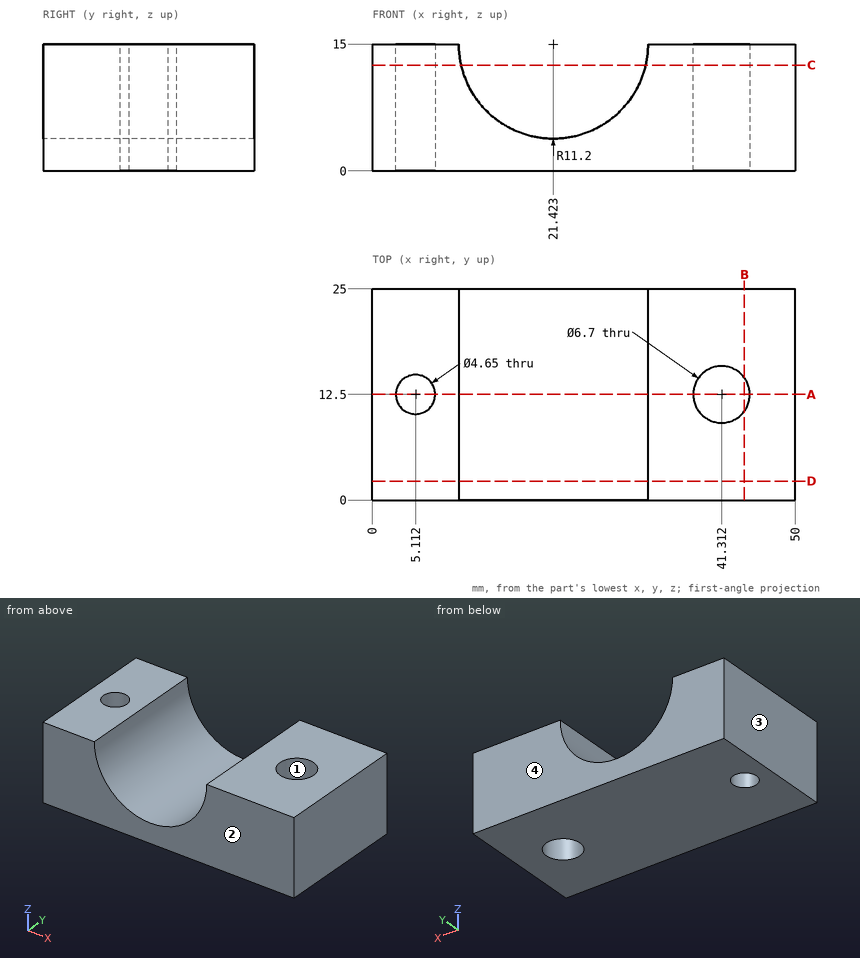
Can you work these out from the drawing? Everything is in mm from the part's minimum corner. Round coordinates to 2 decimals unless told otherwise and drop trailing zeros. Loops run counter-clockwise (first coordinate to the right, second up) from the corner with the lowest first, then second, coordinate; pieces in that order, holes last. Notation, with made-up numbers: (52.25, -18) - (61.25, -18) arc R22 cw to (61.25, -8) - close; hole circle Ø7 at (55.25, 29.5). An arc over 180 degrees is marked (long way). Answer in a Markdown table with one row per item. Add a question column.
(1) If we section it at D-D (y = 2.25): Please give me the cut outline in (x, z), plus the area to 3 significant figures.
(2) If we section it at C-C (z = 12.5): State how many separate pieces and enclosed holes the cut face has, plus the area to 3 significant figures.
(3) If we section it at A-A (y = 12.5): Please give me the cut outline in (x, z), plus the area to 3 significant figures.
(4) If we section it at B-B (x = 44): Please give me the cut outline in (y, z).
(5) If we mould it in two halves opening along Y, with no side actions, what happens to the marked faces 1, 2, 3 and 4? For each: pulls with the +Y half, pulls with the -Y half, needs draft (parallel to the pull), parting line crosses it, or undercut.
(6) I'm going to push a flat-ended pin straight in: pin 1 (4 mm diameter, centred on x = 5.11, y = 12.5, fed in from -Z). Where does the tip first touch, or does it pass through?
(7) I need wall thicknesses on line 1 along Y through (x, z) = (41.5, 12.25) (1 decimal); line 2 along X through (y, z) = (15.5, 9.75) (1 decimal); line 3 along X through (y, z) = (14.5, 9.5) (1 decimal). Which ranges of each line are inside material? Lowest first, please.
Model answer:
| question | item | result |
|---|---|---|
| 1 | outline | (0, 0) - (50, 0) - (50, 15) - (32.62, 15) arc R11.2 cw to (10.22, 15) - (0, 15) - close |
| 1 | area | 553 mm² |
| 2 | separate pieces | 2 |
| 2 | enclosed holes | 2 |
| 2 | area | 652 mm² |
| 3 | outline | (0, 0) - (2.79, 0) - (2.79, 15) - (0, 15) - close; (7.44, 0) - (37.96, 0) - (37.96, 15) - (32.62, 15) arc R11.2 cw to (10.22, 15) - (7.44, 15) - close; (44.66, 0) - (50, 0) - (50, 15) - (44.66, 15) - close |
| 3 | area | 383 mm² |
| 4 | outline | (0, 0) - (10.5, 0) - (10.5, 15) - (0, 15) - close; (14.5, 0) - (25, 0) - (25, 15) - (14.5, 15) - close |
| 5 | face 1 | undercut |
| 5 | face 2 | pulls with the -Y half |
| 5 | face 3 | needs draft |
| 5 | face 4 | pulls with the +Y half |
| 6 | pin 1 | passes through |
| 7 | line 1 | y = 0 to 9.2, 15.8 to 25 |
| 7 | line 2 | x = 0 to 11.5, 31.3 to 39.8, 42.8 to 50 |
| 7 | line 3 | x = 0 to 3.9, 6.3 to 11.7, 31.2 to 38.6, 44 to 50 |
